```python
from build123d import *

# Parameters (mm, degrees)
SKETCH2_R          = 5
CUT_EXTRUDE1_DEPTH = 12
CIRPATTERN1_COUNT  = 8


with BuildPart() as part:
    # Sketch1 → Revolve1 (revolve)
    with BuildSketch(Plane(origin=(0, 0, 0), x_dir=(1, 0, 0), z_dir=(0, 1, 0))):
        Polygon((7, 0), (7, 14), (15, 14), (15, 11), (35, 11), (35, 14), (50, 14), (50, 0), align=None)
    revolve(axis=Axis((0, 0, -184.045185168), (0, 0, 1)))

    # Sketch2 → Cut-Extrude1 (cut, through all)
    with BuildSketch(Plane(origin=(0, 0, -11), x_dir=(-1, 0, 0), z_dir=(0, 0, -1))):
        with Locations((0, -25)):
            Circle(SKETCH2_R)
    cut_extrude1 = extrude(amount=-CUT_EXTRUDE1_DEPTH, mode=Mode.SUBTRACT)

    # CirPattern1: Cut-Extrude1 ×8 about axis
    cirpattern1_axis = Axis((0, 0, 0), (0, 0, 1))
    for i in range(1, CIRPATTERN1_COUNT):
        add(cut_extrude1.rotate(cirpattern1_axis, i * 360 / CIRPATTERN1_COUNT), mode=Mode.SUBTRACT)

    # Mirror1: part across plane


with BuildPart() as part_1:
    add(part.part)
    add(part.part.mirror(Plane.XY))


solid = part_1.part
```
Here's how the part is built. I have some questions about the finished solid (model axes, mm). A direction names the side the tool comes from. Coordinates: 2 decimals unless noted, no trailing zeros. Write each loop counter-clockwise with the first axis right and the second up, starting at its lowest first coordinate (ties: lowest second). Pieces come first, ordered by that corner, then holes. Notation, with made-up numbers: M -39,16.25 L -6,16.25 A32 ccw -6,43.25 Z; hole C 85.25,74 d3. An arc over 180 degrees is marked long. Answer as CSV lines item,"result". Start each with the question number.
Q1. For faces 4 (the cylindrical face through (-14.985, 0.66, -12.479)), 5 (the cylindrical face through (22.446, 19.183, 0.154)), 6 (the cylindrical face through (-28, -21, 13)), which set-ups out of +Z, -Z, +X, -X, +Y, -Y let a thin tool reach every point of the face, with its end or its side?
Q2. Suppose I cut it at A-A, the plane x = 0. State how many separate pieces and enclosed holes the cut face has, then the cut area to 3 significant figures.
Q3. Will these pins go through, and if not, where does the flat tip stop? pin 1 Ø1.5 at (x, z) = (7.5, 9.5) entering from -Y; pin 2 Ø10 at (x, z) = (0, -3.5) entering from +Y; pin 3 Ø6 at (x, y) = (-25, 0) entering from +Z; pin 4 Ø6 at (y, z) = (-5, 5) entering from -X.
Q4. Suppose I cut it at B-B, the plane y = -25. List the corners of the cut face in (x, z) for me, then the cut area to 3 significant figures.
Q5. Suppose I cut it at C-C, the plane z = 12.25. List the corners of the cut face in (x, y) for me.
Q6. If we mould it in two halves opening along Y, with no side actions, what happens to faces 1 (the cylindrical face through (-28, -21, -13)), 2 (the cylindrical face through (19.183, -22.446, 0.154)), 3 (the flat face through (-3.1, -6.5, -14))? For each: pulls with the +Y half, pulls with the -Y half, needs draft (parallel to the pull), parting line crosses it, or undercut.
Q7. I need wall thicknesses on probe 1 along Y at (x, z) = (0, -6.75); probe 2 along X at (y, z) = (21, -7); probe 3 along X at (y, z) = (-15, -6.5). Which ranges of each line are inside material? Lowest first, please. Write a range as [from, to].
Entries:
1,face 4,"-Z"
1,face 5,"+Z, -Z"
1,face 6,"+Z"
2,separate pieces,"4"
2,enclosed holes,"0"
2,area,"1,730 mm²"
3,pin 1,"stops at y = -49.54"
3,pin 2,"stops at y = 50"
3,pin 3,"passes through"
3,pin 4,"stops at x = -49.96"
4,outline,"M -43.3,-14 L -24.49,-14 L -24.49,-11 L -5,-11 L -5,11 L -24.49,11 L -24.49,14 L -43.3,14 Z; M 5,-11 L 24.49,-11 L 24.49,-14 L 43.3,-14 L 43.3,14 L 24.49,14 L 24.49,11 L 5,11 Z"
4,area,"1,910 mm²"
5,outline,"C 0,0 d100; C 0,0 d30; hole C 0,0 d70; hole C 0,0 d14"
6,face 1,"undercut"
6,face 2,"undercut"
6,face 3,"needs draft"
7,probe 1,"y = [-50, -30], [-20, -7], [7, 20], [30, 50]"
7,probe 2,"x = [-45.38, -21.41], [-13.94, -3], [3, 13.94], [21.41, 45.38]"
7,probe 3,"x = [-47.7, -21.9], [-13.46, 13.46], [21.9, 47.7]"
